The model under review builds one solid part; all positions refer to its coordinate system, in mm. Coordinates: 2 decimals unless noted, no trailing zeros. Order: outer loops, then holes, each group sorted by start corner. A loop starts at its lowest first (then second) coordinate and runs counter-clockwise, first axis right, second up. Notation, with made-up numbers: (14, 5.25) -> (49, 5.25) arc R21 ccw to (49, 11.25) -> close; hole circle Ø11 at (78, 80). An arc over 180 degrees is marked (long way). Use one line per item in the form item = value. Start each with the question number.
(1) Take a section at C-C (z = 97.5). State the section outline as (x, y) points, then the cut area to 3 significant figures.
(2) Take a section at A-A (y = -2.45). State how many separate pieces and enclosed holes the cut face has, then the cut area to 3 significant figures.
(3) Take a section at B-B (x = 51). State the section outline as (y, z) points.
(4) Insertion check: pin 1 Ø1.5 at (x, y) = (266, -1.5) entering from -Z; pin 2 Ø1.5 at (y, z) = (-1.5, 0.5) entering from +X; pin 3 Ø3 at (x, z) = (69.13, 23.61) entering from -Y; pin 4 Ø1.5 at (y, z) = (-2, 89.5) entering from +X. Each pin has a flat end and moves straight along its axis. Give the tip position at first contact, or say it passes through.
(5) Wall thickness on line 1 along X through (y, z) = (-2.2, 57.5); line 2 along Z through (x, y) = (131, -0.3); line 3 along Z through (x, y) = (291, -0.5): over which ranges is each line inside the solid? List them lowest first.
```python
from build123d import *

# Parameters (mm, degrees)
F0_R     = 1.6256
F1_DEPTH = 2.9718


with BuildPart() as f1:
    # F0 (on Front) → F1 (new body)
    with BuildSketch(Plane.XZ):
        with BuildLine():
            ThreePointArc((216.986084, 72.877465), (218.795783, 71.831543), (220.139584, 73.432532))
            ThreePointArc((220.139584, 73.432532), (218.232184, 75.03352), (216.986084, 72.877465))
        make_face()
        with BuildLine():
            ThreePointArc((70.752836, 23.610366), (70.733686, 23.85915), (70.676688, 24.102072))
            ThreePointArc((70.676688, 24.102072), (67.520786, 23.361582), (70.752836, 23.610366))
        make_face()
        with BuildLine():
            Line((260.896319, 144.802258), (25.4, 39.681211))
            Line((25.4, 39.681211), (25.4, 1.581211))
            Line((25.4, 1.581211), (90.4748, 1.581211))
            Line((90.4748, 1.581211), (90.4748, -1.390589))
            Line((90.4748, -1.390589), (115.8748, -1.390589))
            Line((115.8748, -1.390589), (115.8748, 1.581211))
            Line((115.8748, 1.581211), (215.811484, 1.581211))
            Line((215.811484, 1.581211), (215.811484, -1.390589))
            Line((215.811484, -1.390589), (241.227301, -1.390589))
            Line((241.227301, -1.390589), (241.227301, 1.581211))
            Line((241.227301, 1.581211), (310.102867, 1.581211))
            ThreePointArc((310.102867, 1.581211), (334.385206, 89.987396), (260.896319, 144.802258))
        make_face()
        with BuildLine():
            ThreePointArc((70.752836, 23.610366), (67.520786, 23.361582), (70.676688, 24.102072))
            ThreePointArc((70.676688, 24.102072), (70.733686, 23.85915), (70.752836, 23.610366))
        make_face(mode=Mode.SUBTRACT)
        with BuildLine():
            ThreePointArc((96.048958, 32.153762), (96.910351, 34.118272), (98.969804, 33.518311))
            ThreePointArc((98.969804, 33.518311), (99.159165, 33.100022), (99.22401, 32.645468))
            ThreePointArc((99.22401, 32.645468), (97.847193, 31.039018), (96.048958, 32.153762))
        make_face(mode=Mode.SUBTRACT)
        with BuildLine():
            ThreePointArc((113.883712, 43.010474), (114.314419, 45.209093), (116.531911, 44.889469))
            ThreePointArc((116.531911, 44.889469), (116.791034, 44.415764), (116.880706, 43.883316))
            ThreePointArc((116.880706, 43.883316), (115.709659, 42.322561), (113.883712, 43.010474))
        make_face(mode=Mode.SUBTRACT)
        with BuildLine():
            ThreePointArc((129.659065, 55.23398), (130.152459, 57.664507), (132.469333, 56.779638))
            ThreePointArc((132.469333, 56.779638), (132.53827, 56.513791), (132.56147, 56.240133))
            ThreePointArc((132.56147, 56.240133), (131.468318, 54.704205), (129.659065, 55.23398))
        make_face(mode=Mode.SUBTRACT)
        with BuildLine():
            ThreePointArc((144.74166, 62.517484), (146.558763, 63.104845), (147.680459, 61.559317))
            ThreePointArc((147.680459, 61.559317), (146.604455, 60.029441), (144.800882, 60.524852))
            ThreePointArc((144.800882, 60.524852), (144.639337, 60.760022), (144.521396, 61.019812))
            ThreePointArc((144.521396, 61.019812), (144.44656, 61.795852), (144.74166, 62.517484))
        make_face(mode=Mode.SUBTRACT)
        with Locations((291.349751, 20.115141)):
            Circle(F0_R, mode=Mode.SUBTRACT)
        with BuildLine():
            ThreePointArc((184.205659, 61.559317), (185.549459, 63.160306), (187.359158, 62.114383))
            ThreePointArc((187.359158, 62.114383), (187.432248, 61.841117), (187.456859, 61.559317))
            ThreePointArc((187.456859, 61.559317), (185.831259, 59.933717), (184.205659, 61.559317))
        make_face(mode=Mode.SUBTRACT)
        with BuildLine():
            ThreePointArc((216.986084, 72.877465), (218.232184, 75.03352), (220.139584, 73.432532))
            ThreePointArc((220.139584, 73.432532), (218.795783, 71.831543), (216.986084, 72.877465))
        make_face(mode=Mode.SUBTRACT)
    extrude(amount=F1_DEPTH)


solid = f1.part
```
Findings:
q1.outline = (154.93, -2.97) -> (331.38, -2.97) -> (331.38, 0) -> (154.93, 0) -> close
q1.area = 524 mm²
q2.separate_pieces = 1
q2.enclosed_holes = 8
q2.area = 30,600 mm²
q3.outline = (-2.97, 1.58) -> (0, 1.58) -> (0, 51.11) -> (-2.97, 51.11) -> close
q4.pin_1 = 1.58
q4.pin_2 = 241.23
q4.pin_3 = through
q4.pin_4 = 334.8
q5.line_1 = 65.32 to 129.91, 131.96 to 338.57
q5.line_2 = 1.58 to 54.62, 57.86 to 86.82
q5.line_3 = 1.58 to 18.53, 21.7 to 137.65
